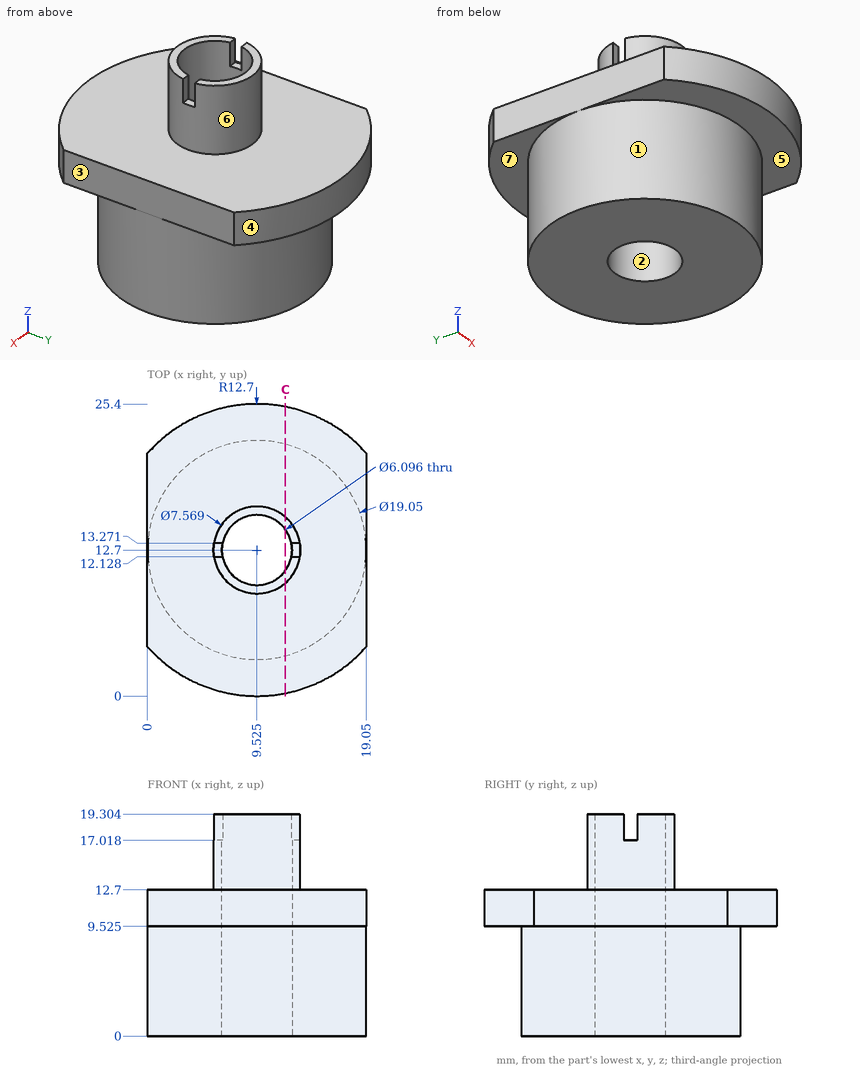
Could you check a few things on this drawing? It's one solid part, dimensions in mm from its lowest x, y, z. A direction names the side the tool comes from. Round coordinates to 2 decimals unless told otherwise and drop trailing zeros. Order: outer loops, then holes, each group sorted by start corner. A loop starts at its lowest first (then second) coordinate and runs counter-clockwise, first axis right, second up. Notation, with made-up numbers: M 52,27 L 59,27 A23 cw 59,45 Z; hole C 11,0 d2. An arc over 180 degrees is marked long. Use a Markdown table: item, result.
1) If I drill on line 1 along X through (y, z) = (12.7, 14.75); line 2 along Z through (x, y) = (11.5, 7.75); line 3 along Z through (x, y) = (4, 22.5) (1 decimal), over which ranges is the centre line in solid material (lowest first)?
Geometry says:
| item | result |
|---|---|
| line 1 | x = 5.74 to 6.48, 12.57 to 13.31 |
| line 2 | z = 0 to 12.7 |
| line 3 | z = 9.5 to 12.7 |
2) On a 3-axis mill with a long thin cutter (end or side, diameter ignored), from which of +Z, -Z, +X, -X, +Y, -Y can I reach the whole of each face in a straight line? I mean the marked faces 4, 5, 6 and 7. Say none if no direction works.
Geometry says:
| item | result |
|---|---|
| face 4 | +Z, -Z, +Y |
| face 5 | -Z, -Y |
| face 6 | +Z |
| face 7 | -Z, +Y |
3) If we mould it in two halves opening along Y, with no side actions, what happens to the marked faces 1, 2 and 3? For each: +Y half, -Y half, draft (parallel to the pull), parting line (faces both ways), or undercut.
Geometry says:
| item | result |
|---|---|
| face 1 | parting line |
| face 2 | undercut |
| face 3 | draft |
4) Imagine slicing it at C-C (x = 12). List the corners of the cut face in (y, z) for me (1 decimal).
Geometry says:
| item | result |
|---|---|
| outline | M 0.2,9.5 L 3.5,9.5 L 3.5,0 L 10.9,0 L 10.9,19.3 L 9.8,19.3 L 9.8,12.7 L 0.2,12.7 Z; M 14.5,0 L 21.9,0 L 21.9,9.5 L 25.2,9.5 L 25.2,12.7 L 15.6,12.7 L 15.6,19.3 L 14.5,19.3 Z |
5) I'm going to push flat-ended pins straight in: P1, Ø2, axis at x = 17, z = 9.5, coming from the -Y side (1 decimal); P2, Ø3, axis at x = 6.5, z = 3, coming from the +Y side; P3, Ø2, axis at x = 3.5, y = 9, coming from the +Z side. Where does each tip first touch, or does it pass through?
Geometry says:
| item | result |
|---|---|
| P1 | stops at y = 1.8 |
| P2 | stops at y = 22.1 |
| P3 | stops at z = 12.7 |
